```python
from build123d import *

# Parameters (mm, degrees)
F0_R     = 26
F0_R_2   = 22.5
F1_DEPTH = 4
F2_DEPTH = 22
F3_T     = -7.5


with BuildPart() as f1:
    # F0 (on Top) → F1 (new body)
    with BuildSketch(Plane.XY):
        Circle(F0_R)
        Circle(F0_R_2, mode=Mode.SUBTRACT)
    extrude(amount=F1_DEPTH)

    # F0 (on Top) → F2 (join)
    with BuildSketch(Plane.XY):
        Circle(F0_R_2)
    extrude(amount=F2_DEPTH)

    # F3
    f3_openings = [f1.faces().sort_by_distance(p)[0] for p in [
        (0, 0, 22),
    ]]
    offset(amount=F3_T, openings=f3_openings)


solid = f1.part
```
The model under review builds one solid part; all positions refer to its coordinate system, in mm. A direction names the side the tool comes from. Coordinates: 2 decimals unless noted, no trailing zeros. Write each loop counter-clockwise with the first axis right and the second up, starting at its lowest first coordinate (ties: lowest second). Pieces come first, ordered by that corner, then holes.
1) Clearance check with flat-ended pins moving along their axes: pin 1 Ø2 at (x, y) = (-8.5, 3) entering from +Z; pin 2 Ø12 at (x, z) = (16.5, 7) entering from -Y; pin 3 Ø5 at (y, z) = (-18.5, 18) entering from -X. State where each tip first meets the part, or that it passes through.
2) Machinability: for faces 1 (the face through (0, 0, 7.5)), 2 (the face through (0, 0, 0)), which of the approach directions +Z, -Z, +X, -X, +Y, -Y give a long, thin tool a straight path to every point of the face, cutting with its end or side? Answer none if there is none.
3) To check wall thickness, follow probe 1 along Y at (x, z) = (0, 16.25); probe 2 along Z at (x, y) = (-0.5, 2.5); probe 3 along Y at (x, z) = (-4, 15). State the ranges of each line that lie inside material, in increasing order.
4) We need section D-D on z = 3. State the section outline as (x, y) points, then the cut area to 3 significant figures.
5) We need section A-A on y = 0. State the section outline as (x, z) points, then the cut area to 3 significant figures.
6) The part is to be moulded in two halves that separate along X. For faces 3 (the face through (15, -5, 22)), 4 (the face through (-14.985, 0.66, 14.648)), 5 (the face through (10.382, -19.961, 12.874)), say which applies: pulls with the +X half, pulls with the -X half, needs draft (parallel to the pull), parting line crosses it, or undercut.
7) We need section C-C on z = 10.5. State the section outline as (x, y) points.
Answer list:
1. pin 1: stops at z = 7.5
1. pin 2: stops at y = -23.41
1. pin 3: stops at x = -15.82
2. face 1: +Z
2. face 2: -Z, +X, -X, +Y, -Y
3. probe 1: y = -22.5 to -15, 15 to 22.5
3. probe 2: z = 0 to 7.5
3. probe 3: y = -22.14 to -14.46, 14.46 to 22.14
4. outline: circle Ø52 at (0, 0)
4. area: 2,120 mm2
5. outline: (-26, 0) - (26, 0) - (26, 4) - (22.5, 4) - (22.5, 22) - (15, 22) - (15, 7.5) - (-15, 7.5) - (-15, 22) - (-22.5, 22) - (-22.5, 4) - (-26, 4) - close
5. area: 583 mm2
6. face 3: needs draft
6. face 4: undercut
6. face 5: parting line crosses it
7. outline: circle Ø45 at (0, 0); hole circle Ø30 at (0, 0)
